```python
from build123d import *

# Parameters (mm, degrees)
SKETCH_3_R      = 2
SKETCH_3_R_2    = 2.08
SKETCH_3_R_3    = 8.75
EXTRUDE_1_DEPTH = 4


with BuildPart() as part:
    # 草图3 → 凸台-拉伸1 (new body)
    with BuildSketch(Plane.XY):
        with BuildLine():
            Line((-38.071041638, 58.740907862), (-46.673377973, 58.740907862))
            ThreePointArc((-46.673377973, 58.740907862), (-46.936210234, 55.880701084), (-47.023930078, 53.009783315))
            Line((-47.023930078, 53.009783315), (-40, -196.990216688))
            ThreePointArc((-40, -196.990216688), (-28.917733212, -224.626509961), (-1.811764706, -236.94916448))
            Line((-1.811764706, -236.94916448), (0, -242.990216688))
            Line((0, -242.990216688), (1.811764706, -236.94916448))
            ThreePointArc((1.811764706, -236.94916448), (28.917733212, -224.626509961), (40, -196.990216688))
            Line((40, -196.990216688), (47.023930078, 53.009783315))
            ThreePointArc((47.023930078, 53.009783315), (46.936210234, 55.880701084), (46.673377973, 58.740907862))
            Line((46.673377973, 58.740907862), (38.071041638, 58.740907862))
            ThreePointArc((38.071041638, 58.740907862), (38.449556599, 54.979960288), (38.457440916, 51.200021389))
            ThreePointArc((38.457440916, 51.200021389), (38.457808554, 37.081210633), (28.474561686, 27.097443846))
            ThreePointArc((28.474561686, 27.097443846), (27.22431994, 25.786881122), (25.913822328, 24.536571126))
            ThreePointArc((25.913822328, 24.536571126), (15.93057546, 14.552804338), (1.811764704, 14.5524367))
            Line((1.811764704, 14.5524367), (-1.811764704, 14.5524367))
            ThreePointArc((-1.811764704, 14.5524367), (-15.93057546, 14.552804338), (-25.913822328, 24.536571126))
            ThreePointArc((-25.913822328, 24.536571126), (-27.22431994, 25.786881122), (-28.474561686, 27.097443846))
            ThreePointArc((-28.474561686, 27.097443846), (-38.457808554, 37.081210633), (-38.457440916, 51.200021389))
            ThreePointArc((-38.457440916, 51.200021389), (-38.449556599, 54.979960288), (-38.071041638, 58.740907862))
        make_face()
        with Locations((0, 10.509783315)):
            Circle(SKETCH_3_R, mode=Mode.SUBTRACT)
        with Locations((-30.0520382, 22.957745114)):
            Circle(SKETCH_3_R, mode=Mode.SUBTRACT)
        with Locations((-42.5, 53.009783315)):
            Circle(SKETCH_3_R, mode=Mode.SUBTRACT)
        with Locations((30.0520382, 22.957745114)):
            Circle(SKETCH_3_R, mode=Mode.SUBTRACT)
        with Locations((0, -211.990216688)):
            Circle(SKETCH_3_R, mode=Mode.SUBTRACT)
        with Locations((-12.990381057, -204.490216688)):
            Circle(SKETCH_3_R, mode=Mode.SUBTRACT)
        with Locations((-12.990381057, -189.490216688)):
            Circle(SKETCH_3_R, mode=Mode.SUBTRACT)
        with Locations((0, -181.990216688)):
            Circle(SKETCH_3_R, mode=Mode.SUBTRACT)
        with Locations((12.990381057, -189.490216688)):
            Circle(SKETCH_3_R, mode=Mode.SUBTRACT)
        with Locations((12.990381057, -204.490216688)):
            Circle(SKETCH_3_R, mode=Mode.SUBTRACT)
        with Locations((-13.53, -196.990216688)):
            Circle(SKETCH_3_R_2, mode=Mode.SUBTRACT)
        with Locations((6.765, -185.272892975)):
            Circle(SKETCH_3_R_2, mode=Mode.SUBTRACT)
        with Locations((6.765, -208.707540401)):
            Circle(SKETCH_3_R_2, mode=Mode.SUBTRACT)
        with Locations((0, -196.990216688)):
            Circle(SKETCH_3_R_3, mode=Mode.SUBTRACT)
        with Locations(Location((42.5, 53.009783315, 0), (0, 0, 180))):
            Circle(SKETCH_3_R, mode=Mode.SUBTRACT)
        with BuildLine():
            Line((-14, -153.564151609), (-14, -15.006038041))
            ThreePointArc((-14, -15.006038041), (0, -1.006038041), (14, -15.006038041))
            Line((14, -15.006038041), (14, -153.564151609))
            ThreePointArc((14, -153.564151609), (0, -167.564151609), (-14, -153.564151609))
        make_face(mode=Mode.SUBTRACT)
    extrude(amount=EXTRUDE_1_DEPTH)


solid = part.part
```
For this review, take the finished solid that the model builds, in its own axes (mm). A direction names the side the tool comes from. Round coordinates to 2 decimals unless told otherwise and drop trailing zeros. Loops run counter-clockwise (first coordinate to the right, second up) from the corner with the lowest first, then second, coordinate; pieces in that order, holes last.
(1) Mouldability with a two-part tool opening along Y and no side actions: class faces 3 (the cylindrical face through (28.621, -224.934, 1.972)), 4 (the cylindrical face through (-15.743, 14.476, 1.972)), 5 (the cylindrical face through (38.534, 37.269, 1.972)) as released by +Y, released by -Y, zero draft, split by the parting line, or undercut.
Returned:
face 3: released by -Y
face 4: released by +Y
face 5: undercut
(2) Tool access review of faces 1 (the cylindrical face through (-0.31, -1.01, 1.97)), 2 (the cylindrical face through (-29.21, -224.32, 1.97)): name each direction out of +Z, -Z, +X, -X, +Y, -Y from which nothing blocks a thin tool from reaching the whole face with its end or side.
Returned:
face 1: +Z, -Z
face 2: +Z, -Z, -X, -Y
(3) We need section D-D (z = 2.2). State how many separate pieces and enclosed holes the cut face has, plus the area to 3 significant figures.
Returned:
separate pieces: 1
enclosed holes: 16
area: 16,900 mm2
(4) We need section A-A (y = -145). Give the boundary of the cut face in (x, z).
Returned:
outline: (-41.46, 0) - (-14, 0) - (-14, 4) - (-41.46, 4) - close; (14, 0) - (41.46, 0) - (41.46, 4) - (14, 4) - close
(5) Clearance check with flat-ended pins moving along their axes: P1, Ø3.5, axis at x = 30.05, y = 22.96, coming from the -Z side; P2, Ø2, axis at y = -131, z = 1.5, coming from the +X side; P3, Ø2, axis at x = -9, z = 3, coming from the -Y side; P4, Ø1.8, axis at x = -1, z = 1.5, coming from the +Y side. State where each tip first meets the part, or that it passes through.
Returned:
P1: passes through
P2: stops at x = 41.88
P3: stops at y = -236.18
P4: stops at y = 14.55
(6) We need section C-C (y = -23). Give the boundary of the cut face in (x, z).
Returned:
outline: (-44.89, 0) - (-14, 0) - (-14, 4) - (-44.89, 4) - close; (14, 0) - (44.89, 0) - (44.89, 4) - (14, 4) - close
(7) Wall thickness on line 1 along X through (y, z) = (-203, 1.5); line 2 along Y through (x, z) = (5.5, 3.85); line 3 along X through (y, z) = (-35, 2.75): over which ranges is each line inside the solid? List them lowest first.
Returned:
line 1: x = -39.55 to -14.32, -11.66 to -6.36, 6.36 to 11.66, 14.32 to 39.55
line 2: y = -236.61 to -210.36, -207.06 to -203.8, -190.18 to -186.92, -183.62 to -166.44, -2.13 to 13.46
line 3: x = -44.55 to -14, 14 to 44.55
(8) We need section B-B (x = 35.5). Give the boundary of the cut face in (y, z).
Returned:
outline: (-215.42, 0) - (32.23, 0) - (32.23, 4) - (-215.42, 4) - close
